```python
from build123d import *

# Parameters (mm, degrees)
RESSALTO_EXTRUS_O1_DEPTH = 100


with BuildPart() as part:
    # Esboço1 → Ressalto-extrusão1 (new body, symmetric)
    with BuildSketch(Plane.XY):
        with BuildLine():
            Line((-13.1, 8.9), (-14.2, 10))
            Line((-14.2, 10), (-19.6, 10))
            ThreePointArc((-19.6, 10), (-19.882842712, 9.882842712), (-20, 9.6))
            Line((-20, 9.6), (-20, 4.2))
            Line((-20, 4.2), (-18.9, 3.1))
            ThreePointArc((-18.9, 3.1), (-18.617157287, 3.217157287), (-18.5, 3.5))
            Line((-18.5, 3.5), (-18.5, 5.5))
            Line((-18.5, 5.5), (-16.560660172, 5.5))
            Line((-16.560660172, 5.5), (-14.332233047, 3.271572875))
            ThreePointArc((-14.332233047, 3.271572875), (-13.790301169, 2.460514503), (-13.6, 1.503805922))
            Line((-13.6, 1.503805922), (-13.6, 0))
            Line((-13.6, 0), (-13.6, -1.503805922))
            ThreePointArc((-13.6, -1.503805922), (-13.790301169, -2.460514503), (-14.332233047, -3.271572875))
            Line((-14.332233047, -3.271572875), (-16.560660172, -5.5))
            Line((-16.560660172, -5.5), (-18.5, -5.5))
            Line((-18.5, -5.5), (-18.5, -3.5))
            ThreePointArc((-18.5, -3.5), (-18.617157287, -3.217157288), (-18.9, -3.1))
            Line((-18.9, -3.1), (-20, -4.2))
            Line((-20, -4.2), (-20, -9.6))
            ThreePointArc((-20, -9.6), (-19.882842712, -9.882842712), (-19.6, -10))
            Line((-19.6, -10), (-14.2, -10))
            Line((-14.2, -10), (-13.1, -8.9))
            ThreePointArc((-13.1, -8.9), (-13.217157287, -8.617157288), (-13.5, -8.5))
            Line((-13.5, -8.5), (-15.5, -8.5))
            Line((-15.5, -8.5), (-15.5, -6.560660172))
            Line((-15.5, -6.560660172), (-13.271572875, -4.332233047))
            ThreePointArc((-13.271572875, -4.332233047), (-12.460514503, -3.790301169), (-11.503805922, -3.6))
            Line((-11.503805922, -3.6), (-10, -3.6))
            Line((-10, -3.6), (-8.496194078, -3.6))
            ThreePointArc((-8.496194078, -3.6), (-7.539485497, -3.790301169), (-6.728427125, -4.332233047))
            Line((-6.728427125, -4.332233047), (-4.5, -6.560660172))
            Line((-4.5, -6.560660172), (-4.5, -8.5))
            Line((-4.5, -8.5), (-6.5, -8.5))
            ThreePointArc((-6.5, -8.5), (-6.782842712, -8.617157288), (-6.9, -8.9))
            Line((-6.9, -8.9), (-5.8, -10))
            Line((-5.8, -10), (5.8, -10))
            Line((5.8, -10), (6.9, -8.9))
            ThreePointArc((6.9, -8.9), (6.782842712, -8.617157288), (6.5, -8.5))
            Line((6.5, -8.5), (4.5, -8.5))
            Line((4.5, -8.5), (4.5, -6.560660172))
            Line((4.5, -6.560660172), (6.728427125, -4.332233047))
            ThreePointArc((6.728427125, -4.332233047), (7.539485497, -3.790301169), (8.496194078, -3.6))
            Line((8.496194078, -3.6), (10, -3.6))
            Line((10, -3.6), (11.503805922, -3.6))
            ThreePointArc((11.503805922, -3.6), (12.460514503, -3.790301169), (13.271572875, -4.332233047))
            Line((13.271572875, -4.332233047), (15.5, -6.560660172))
            Line((15.5, -6.560660172), (15.5, -8.5))
            Line((15.5, -8.5), (13.5, -8.5))
            ThreePointArc((13.5, -8.5), (13.217157287, -8.617157288), (13.1, -8.9))
            Line((13.1, -8.9), (14.2, -10))
            Line((14.2, -10), (19.6, -10))
            ThreePointArc((19.6, -10), (19.882842712, -9.882842712), (20, -9.6))
            Line((20, -9.6), (20, -4.2))
            Line((20, -4.2), (18.9, -3.1))
            ThreePointArc((18.9, -3.1), (18.617157287, -3.217157288), (18.5, -3.5))
            Line((18.5, -3.5), (18.5, -5.5))
            Line((18.5, -5.5), (16.560660172, -5.5))
            Line((16.560660172, -5.5), (14.332233047, -3.271572875))
            ThreePointArc((14.332233047, -3.271572875), (13.790301169, -2.460514503), (13.6, -1.503805922))
            Line((13.6, -1.503805922), (13.6, 0))
            Line((13.6, 0), (13.6, 1.503805922))
            ThreePointArc((13.6, 1.503805922), (13.790301169, 2.460514503), (14.332233047, 3.271572875))
            Line((14.332233047, 3.271572875), (16.560660172, 5.5))
            Line((16.560660172, 5.5), (18.5, 5.5))
            Line((18.5, 5.5), (18.5, 3.5))
            ThreePointArc((18.5, 3.5), (18.617157287, 3.217157287), (18.9, 3.1))
            Line((18.9, 3.1), (20, 4.2))
            Line((20, 4.2), (20, 9.6))
            ThreePointArc((20, 9.6), (19.882842712, 9.882842712), (19.6, 10))
            Line((19.6, 10), (14.2, 10))
            Line((14.2, 10), (13.1, 8.9))
            ThreePointArc((13.1, 8.9), (13.217157287, 8.617157287), (13.5, 8.5))
            Line((13.5, 8.5), (15.5, 8.5))
            Line((15.5, 8.5), (15.5, 6.560660172))
            Line((15.5, 6.560660172), (13.271572875, 4.332233047))
            ThreePointArc((13.271572875, 4.332233047), (12.460514503, 3.790301169), (11.503805922, 3.6))
            Line((11.503805922, 3.6), (10, 3.6))
            Line((10, 3.6), (8.496194078, 3.6))
            ThreePointArc((8.496194078, 3.6), (7.539485497, 3.790301169), (6.728427125, 4.332233047))
            Line((6.728427125, 4.332233047), (4.5, 6.560660172))
            Line((4.5, 6.560660172), (4.5, 8.5))
            Line((4.5, 8.5), (6.5, 8.5))
            ThreePointArc((6.5, 8.5), (6.782842712, 8.617157288), (6.9, 8.9))
            Line((6.9, 8.9), (5.8, 10))
            Line((5.8, 10), (-5.8, 10))
            Line((-5.8, 10), (-6.9, 8.9))
            ThreePointArc((-6.9, 8.9), (-6.782842712, 8.617157288), (-6.5, 8.5))
            Line((-6.5, 8.5), (-4.5, 8.5))
            Line((-4.5, 8.5), (-4.5, 6.560660172))
            Line((-4.5, 6.560660172), (-6.728427125, 4.332233047))
            ThreePointArc((-6.728427125, 4.332233047), (-7.539485497, 3.790301169), (-8.496194078, 3.6))
            Line((-8.496194078, 3.6), (-10, 3.6))
            Line((-10, 3.6), (-11.503805922, 3.6))
            ThreePointArc((-11.503805922, 3.6), (-12.460514503, 3.790301169), (-13.271572875, 4.332233047))
            Line((-13.271572875, 4.332233047), (-15.5, 6.560660172))
            Line((-15.5, 6.560660172), (-15.5, 8.5))
            Line((-15.5, 8.5), (-13.5, 8.5))
            ThreePointArc((-13.5, 8.5), (-13.217157287, 8.617157287), (-13.1, 8.9))
        make_face()
        with BuildLine():
            Line((-3, 8.5), (3, 8.5))
            Line((3, 8.5), (3, 6.105025253))
            ThreePointArc((3, 6.105025253), (3.030448187, 5.95195188), (3.117157288, 5.822182541))
            Line((3.117157288, 5.822182541), (5.667766953, 3.271572875))
            ThreePointArc((5.667766953, 3.271572875), (6.209698831, 2.460514503), (6.4, 1.503805922))
            Line((6.4, 1.503805922), (6.4, 0))
            Line((6.4, 0), (6.4, -1.503805922))
            ThreePointArc((6.4, -1.503805922), (6.209698831, -2.460514503), (5.667766953, -3.271572875))
            Line((5.667766953, -3.271572875), (3.117157288, -5.822182541))
            ThreePointArc((3.117157288, -5.822182541), (3.030448187, -5.95195188), (3, -6.105025253))
            Line((3, -6.105025253), (3, -8.5))
            Line((3, -8.5), (-3, -8.5))
            Line((-3, -8.5), (-3, -6.105025253))
            ThreePointArc((-3, -6.105025253), (-3.030448187, -5.95195188), (-3.117157288, -5.822182541))
            Line((-3.117157288, -5.822182541), (-5.667766953, -3.271572875))
            ThreePointArc((-5.667766953, -3.271572875), (-6.209698831, -2.460514503), (-6.4, -1.503805922))
            Line((-6.4, -1.503805922), (-6.4, 0))
            Line((-6.4, 0), (-6.4, 1.503805922))
            ThreePointArc((-6.4, 1.503805922), (-6.209698831, 2.460514503), (-5.667766953, 3.271572875))
            Line((-5.667766953, 3.271572875), (-3.117157288, 5.822182541))
            ThreePointArc((-3.117157288, 5.822182541), (-3.030448187, 5.95195188), (-3, 6.105025253))
            Line((-3, 6.105025253), (-3, 8.5))
        make_face(mode=Mode.SUBTRACT)
        with BuildLine():
            ThreePointArc((-10, 2.5), (-11.767766953, 1.767766953), (-12.5, 0))
            ThreePointArc((-12.5, 0), (-11.767766953, -1.767766953), (-10, -2.5))
            ThreePointArc((-10, -2.5), (-8.232233047, -1.767766953), (-7.5, 0))
            ThreePointArc((-7.5, 0), (-8.232233047, 1.767766953), (-10, 2.5))
        make_face(mode=Mode.SUBTRACT)
        with BuildLine():
            ThreePointArc((12.5, 0), (11.767766953, -1.767766953), (10, -2.5))
            ThreePointArc((10, -2.5), (8.232233047, -1.767766953), (7.5, 0))
            ThreePointArc((7.5, 0), (8.232233047, 1.767766953), (10, 2.5))
            ThreePointArc((10, 2.5), (11.767766953, 1.767766953), (12.5, 0))
        make_face(mode=Mode.SUBTRACT)
    extrude(amount=RESSALTO_EXTRUS_O1_DEPTH, both=True)


solid = part.part
```
The model under review builds one solid part; all positions refer to its coordinate system, in mm. Give positions to 0.01 mm unless a question says otherwise; leave off trailing zeros.
(1) For P1, Ø0.9, axis at y = -0.5, z = -37.5, coming from the +X side; P2, Ø10, axis at x = 6.5, z = -64.5, coming from the +Y side; P3, Ø3.5, axis at y = -0.5, z = -32, coming from the -X side; P4, Ø4, axis at y = 2, z = 51.5, coming from the -X side, all flat-tipped, find the tip position at first contact; note any pin that passes through.
(2) Consider section A-A, the plane z = 22. Give the number of separate pieces and of enclosed holes in the cut face, and give its area (3 significant figures).
(3) To check wall thickness, follow L1, parallel to X at y = 7.25, z = -10.5; L2, parallel to X at y = 4.5, z = 11; L3, parallel to Y at x = 0.5, z = 57. State the ranges of each line that lie inside material, in increasing order.
Returned:
1. P1: stops at x = 13.6
1. P2: stops at y = 10
1. P3: stops at x = -13.71
1. P4: stops at x = -19.8
2. separate pieces: 1
2. enclosed holes: 3
2. area: 269 mm2
3. L1: x = -20 to -15.5, -4.5 to -3, 3 to 4.5, 15.5 to 20
3. L2: x = -20 to -18.5, -15.56 to -13.44, -6.56 to -4.44, 4.44 to 6.56, 13.44 to 15.56, 18.5 to 20
3. L3: y = -10 to -8.5, 8.5 to 10
